Autodesk Inventor part; units mm, degrees
ref_plane "YZ Plane" through (0, 0, 0) normal (1, 0, 0) x (0, 1, 0)
ref_plane "XZ Plane" through (0, 0, 0) normal (0, 1, 0) x (-1, 0, 0)
ref_plane "XY Plane" through (0, 0, 0) normal (0, 0, 1) x (1, 0, 0)
sketch "Sketch1" plane through (0, 0, 0) normal (1, 0, 0) x (0, 1, 0)
  line L0 (-25.4, -50.8) -> (25.4, -50.8)
  line L1 (25.4, -50.8) -> (25.4, 50.8)
  line L2 (25.4, 50.8) -> (-25.4, 50.8)
  line L3 (-25.4, 50.8) -> (-25.4, -50.8)
  line L4 (-25.4, -50.8) -> (25.4, 50.8) construction
  line L5 (25.4, -50.8) -> (-25.4, 50.8) construction
  point P0 (0, 0)
  dimension "d0" = 50.8
  dimension "d1" = 101.6
extrude "Extrusion1" add sketch "Sketch1" along normal blind 44.45
fillet "Fillet2" radius 9.525 4 edges at (22.225, 25.4, 50.8) (22.225, -25.4, 50.8) (22.225, -25.4, -50.8) (22.225, 25.4, -50.8)
sketch "Sketch5" plane through (44.45, 0, 0) normal (1, 0, 0) x (0, 0, -1)
  arc A0 (50.8, 15.875) -> (41.275, 25.4) centre (41.275, 15.875) ccw
  line L0 (41.275, 25.4) -> (-41.275, 25.4)
  arc A1 (-41.275, 25.4) -> (-50.8, 15.875) centre (-41.275, 15.875) ccw
  line L1 (-50.8, 15.875) -> (-50.8, -15.875)
  arc A2 (-50.8, -15.875) -> (-41.275, -25.4) centre (-41.275, -15.875) ccw
  line L2 (-41.275, -25.4) -> (41.275, -25.4)
  arc A3 (41.275, -25.4) -> (50.8, -15.875) centre (41.275, -15.875) ccw
  line L3 (50.8, -15.875) -> (50.8, 15.875)
  point P0 (0, 0)
hole "Hole2" at (44.45, -15.875, -41.275) at (44.45, -15.875, 41.275) at (44.45, 15.875, 41.275) at (44.45, 15.875, -41.275) direction (-1, 0, 0) diameter 6.7564 end through all
sketch "Sketch6" plane through (44.45, 0, 0) normal (1, 0, 0) x (0, 0, -1)
  circle A0 centre (41.275, -15.875) radius 3.3782
  circle A1 centre (41.275, -15.875) radius 6.985
  circle A2 centre (41.275, 15.875) radius 3.3782
  circle A3 centre (41.275, 15.875) radius 6.985
  circle A4 centre (-41.275, 15.875) radius 3.3782
  circle A5 centre (-41.275, 15.875) radius 6.985
  circle A6 centre (-41.275, -15.875) radius 3.3782
  circle A7 centre (-41.275, -15.875) radius 6.985
  line L0 (-48.26, 22.86) -> (48.26, 22.86)
  line L1 (48.26, 22.86) -> (48.26, -22.86)
  line L2 (48.26, -22.86) -> (-48.26, -22.86)
  line L3 (-48.26, -22.86) -> (-48.26, 22.86)
  line L4 (-48.26, 22.86) -> (48.26, -22.86) construction
  line L5 (48.26, 22.86) -> (-48.26, -22.86) construction
  arc A8 (41.275, -25.4) -> (50.8, -15.875) centre (41.275, -15.875) ccw
  arc A9 (50.8, 15.875) -> (41.275, 25.4) centre (41.275, 15.875) ccw
  arc A10 (-41.275, 25.4) -> (-50.8, 15.875) centre (-41.275, 15.875) ccw
  arc A11 (-50.8, -15.875) -> (-41.275, -25.4) centre (-41.275, -15.875) ccw
  line L6 (50.8, -15.875) -> (50.8, 15.875)
  line L7 (41.275, 25.4) -> (-41.275, 25.4)
  point P0 (0, 0)
  point P1 (-48.26, 15.875)
  point P2 (-48.26, -15.875)
  point P3 (-41.275, -22.86)
  point P4 (41.275, -22.86)
  point P5 (48.26, -15.875)
  point P6 (48.26, 15.875)
  point P7 (41.275, 22.86)
  point P8 (-41.275, 22.86)
  dimension "d24" = 2.54
  dimension "d27" = 2.54
extrude "Extrusion2" cut sketch "Sketch6" against normal through all contours A1 L2 A7 L3 A5 L0 A3 L1
fillet "Fillet3" radius 6.35 8 edges at (22.225, 15.875, 48.26) (22.225, 22.86, 41.275) (22.225, -22.86, -41.275) (22.225, -15.875, -48.26) (22.225, 15.875, -48.26) (22.225, 22.86, -41.275) (22.225, -22.86, 41.275) (22.225, -15.875, 48.26)
equation "\"d2\" = Base"
equation "\"Base\" = 44.45"
properties part number "NASA-20-MM-MB-01" material "Aluminum 6061"
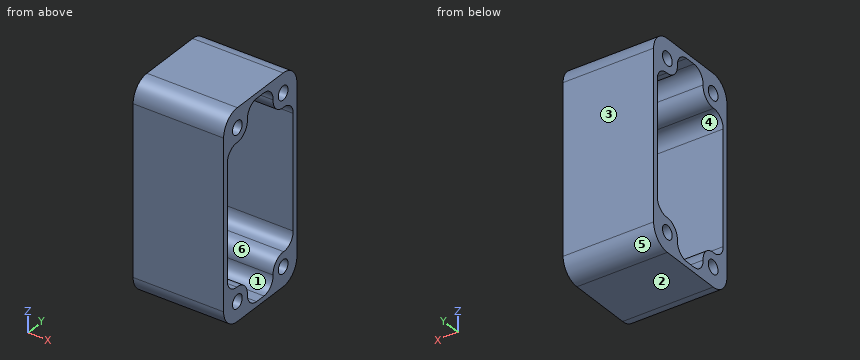
The model under review builds one solid part; all positions refer to its coordinate system, in mm. Face numbers are marked on the shaded views. A direction names the side the tool comes from. Round coordinates to 2 decimals unless told otherwise and drop trailing zeros. Loops run counter-clockwise (first coordinate to the right, second up) from the corner with the lowest first, then second, coordinate; pieces in that order, holes last. Notation, with made-up numbers: (61, 48.5) - (102, 48.5) arc R20 ccw to (102, 65.5) - close; hole circle Ø8 at (-13, 65.5). An arc over 180 degrees is marked (long way). Write each question's results on one line, items separated by ' | '. Start each with the question number.
Q1. Tool access review of the marked faces 1 and 2: name each direction out of +Z, -Z, +X, -X, +Y, -Y from which nothing blocks a thin tool from reaching the whole face with its end or side.
Q2. Take a section at C-C on x = 28.5. Give the number of separate pieces and of enclosed holes in the cut face, plus the area to 3 significant figures.
Q3. Wall thickness on line 1 along Z through (x, y) = (24.5, -16); line 2 along Z through (x, y) = (4.5, -1); line 3 along Y through (x, z) = (24, 41): over which ranges is each line inside the solid? List them lowest first. Write a range as [from, to].
Q4. Take a section at A-A on z = -16. Give the boundary of the cut face in (x, y), plus the area to 3 significant figures.
Q5. Draft analysis for pull direction Z (two halves, no side actions). For the marked faces 3, 4, 5 and 6, state which applies: pulls with the +Z half, pulls with the -Z half, needs draft (parallel to the pull), parting line crosses it, or undercut.
Q6. Take a section at B-B on y = 11. Give the boundary of the cut face in (x, z), plus the area to 3 significant figures.
Data:
1) face 1: +X, -X | face 2: -Z, +X, -X, +Y, -Y
2) separate pieces: 1 | enclosed holes: 5 | area: 1,330 mm²
3) line 1: z = [-50.8, -44.65], [-37.9, -34.29], [34.29, 37.9], [44.65, 50.8] | line 2: z = [-50.8, -48.26], [48.26, 50.8] | line 3: y = [-25.4, -19.24], [-12.51, -8.9], [8.9, 12.51], [19.24, 25.4]
4) outline: (0, -25.4) - (44.45, -25.4) - (44.45, -22.86) - (0, -22.86) - close; (0, 22.86) - (44.45, 22.86) - (44.45, 25.4) - (0, 25.4) - close | area: 226 mm²
5) face 3: needs draft | face 4: undercut | face 5: pulls with the -Z half | face 6: undercut
6) outline: (0, -50.8) - (44.45, -50.8) - (44.45, -36.27) - (0, -36.27) - close; (0, 36.27) - (44.45, 36.27) - (44.45, 50.8) - (0, 50.8) - close | area: 1,290 mm²
